Could you check a few things on this model? Use its own coordinates, in mm. Face numbers are marked on the shaded views. A direction names the side the tool comes from. Round coordinates to 2 decimals unless told otherwise and drop trailing zeros. Loops run counter-clockwise (first coordinate to the right, second up) from the corner with the lowest first, then second, coordinate; pieces in that order, holes last. Notation, with made-up numbers: M 84,-37.75 L 88,-37.75 A10 ccw 88,-30.75 Z; hole C 11,81 d8. An arc over 180 degrees is marked long. One line per item, written item: value. Start each with the question number.
Q1. I'm going to push flat-ended pins straight in: pin 1 Ø6.5 at (y, z) = (0, 6) entering from +X; pin 2 Ø6 at (y, z) = (0, 20) entering from -X; pin 3 Ø4.5 at (x, y) = (3, -3) entering from +Z. Where does each tip first touch, or does it pass through?
Q2. Imagine slicing it at A-A (y = 0). Give the number of separate pieces and of enclosed holes in the cut face, then the cut area to 3 significant figures.
Q3. Which directions (+Z, -Z, +X, -X, +Y, -Y) give clear straight access to the entire face, cutting with the end or side of a thin tool? Please do the marked faces 4 and 5.
Q4. Thinking about a two-plate mould opening in X: for the marked faces 1, 2 and 3, which applies, released by +X, released by -X, zero draft, split by the parting line, or undercut?
Q5. Imagine slicing it at D-D (z = 12.5). Please give me the cut outline in (x, y), then the cut area to 3 significant figures.
Q6. Please list where these lines run through material, in increasing order: line 1 along Z through (x, y) = (1.75, 0); line 2 along Y through (x, z) = (3.5, 20); line 3 along Z through (x, y) = (2.5, -0.5).
Q7. Imagine slicing it at C-C (x = 0). Please give me the cut outline in (y, z).
Q8. Imagine slicing it at B-B (z = 20). Please give me the cut outline in (x, y).
from build123d import *

# Parameters (mm, degrees)
F0_W           = 20
F0_H           = 20
F1_DEPTH       = 35
F2_R           = 7.7
F3_DEPTH       = 8.5
F5_D           = 5
F5_CSINK_D     = 9.8
F5_CSINK_ANGLE = 90
F6_R           = 5
F7_SIZE        = 0.8


with BuildPart() as f1:
    # F0 (on Top) → F1 (new body)
    with BuildSketch(Plane.XY):
        Rectangle(F0_W, F0_H)
    extrude(amount=F1_DEPTH)

    # F2 (on face) → F3 (cut)
    with BuildSketch(Plane.XY.offset(35)):
        Circle(F2_R)
    extrude(amount=-F3_DEPTH, mode=Mode.SUBTRACT)

    # F5 (through all)
    with Locations(Plane(origin=(-10, 0, 0), x_dir=(0, -1, 0), z_dir=(-1, 0, 0))):
        with Locations((0, 6), (0, 20)):
            CounterSinkHole(F5_D / 2, F5_CSINK_D / 2, counter_sink_angle=F5_CSINK_ANGLE)

    # F6
    f6_edges = [f1.edges().sort_by_distance(p)[0] for p in [
        (-10, -10, 17.5),
        (-10, 10, 17.5),
    ]]
    fillet(f6_edges, radius=F6_R)

    # F7
    f7_edges = [f1.edges().sort_by_distance(p)[0] for p in [
        (-7.7, 0, 35),
        (10, -10, 17.5),
        (10, 10, 17.5),
        (2.5, 10, 35),
        (-10, 0, 35),
        (10, 0, 35),
        (-10, 0, 0),
        (2.5, 10, 0),
        (10, 0, 0),
        (2.5, -10, 0),
        (2.5, -10, 35),
        (-8.535534, -8.535534, 0),
        (-8.535534, 8.535534, 0),
        (-8.535534, -8.535534, 35),
        (10, 2.5, 20),
        (10, 2.5, 6),
        (-8.535534, 8.535534, 35),
    ]]
    chamfer(f7_edges, length=F7_SIZE)


solid = f1.part
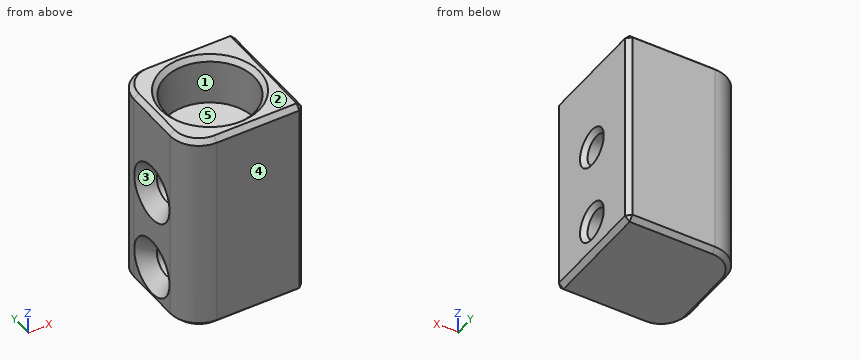
Report:
1. pin 1: stops at x = 9.95
1. pin 2: stops at x = -8.1
1. pin 3: stops at z = 26.5
2. separate pieces: 3
2. enclosed holes: 0
2. area: 354 mm²
3. face 4: +Z, -Z, +X, -X, -Y
3. face 5: +Z
4. face 1: undercut
4. face 2: zero draft
4. face 3: released by -X
5. outline: M -10,-5 A5 ccw -5,-10 L 9.2,-10 L 10,-9.2 L 10,9.2 L 9.2,10 L -5,10 A5 ccw -10,5 Z
5. area: 389 mm²
6. line 1: z = 0 to 3.5, 8.5 to 17.5, 22.5 to 26.5
6. line 2: y = -10 to -2.5, 2.5 to 10
6. line 3: z = 0 to 3.55, 8.45 to 17.55, 22.45 to 26.5
7. outline: M -10,0.8 L -9.2,0 L 9.2,0 L 10,0.8 L 10,34.2 L 9.2,35 L 8.5,35 L 7.7,34.2 L 7.7,26.5 L -7.7,26.5 L -7.7,34.2 L -8.5,35 L -9.2,35 L -10,34.2 Z; hole C 0,6 d5; hole C 0,20 d5
8. outline: M -10,-5 A5 ccw -5,-10 L 9.2,-10 L 10,-9.2 L 10,-3.3 L 9.2,-2.5 L -7.6,-2.5 L -10,-4.9 Z; M -10,4.9 L -7.6,2.5 L 9.2,2.5 L 10,3.3 L 10,9.2 L 9.2,10 L -5,10 A5 ccw -10,5 Z
